```python
from build123d import *

# Parameters (mm, degrees)
F0_R     = 11
F1_DEPTH = 2.5
F2_SIZE  = 1.016
F3_R     = 8.25
F4_DEPTH = 0.5


with BuildPart() as f1:
    # F0 (on Top) → F1 (new body)
    with BuildSketch(Plane.XY):
        Circle(F0_R)
    extrude(amount=F1_DEPTH)

    # F2
    f2_edges = [f1.edges().sort_by_distance(p)[0] for p in [
        (-11, 0, 2.5),
    ]]
    chamfer(f2_edges, length=F2_SIZE)

    # F3 (on face) → F4 (cut)
    with BuildSketch(Plane(origin=(0, 0, 0), x_dir=(1, 0, 0), z_dir=(0, 0, -1))):
        Circle(F3_R)
    extrude(amount=-F4_DEPTH, mode=Mode.SUBTRACT)


solid = f1.part
```
Verification items for the finished model (mm, model axes). A direction names the side the tool comes from. Coordinates: 2 decimals unless noted, no trailing zeros. Loops run counter-clockwise (first coordinate to the right, second up) from the corner with the lowest first, then second, coordinate; pieces in that order, holes last. Notation, with made-up numbers: (81, -3) - (88, -3) arc R14 cw to (88, 6) - close; hole circle Ø4 at (33, 85.5). An arc over 180 degrees is marked (long way). Put each result on its own line as item: value.
Item 1: Section check C-C (z = 0.95). Enter the section's corners in (x, y).
Conclusion:
outline: circle Ø22 at (0, 0)
Item 2: Gauge pin test, flat ends, axial feed: pin 1 Ø1 at (x, z) = (4, 2) entering from +Y; pin 2 Ø1.5 at (x, z) = (-7.5, 1) entering from -Y; pin 3 Ø1.5 at (x, z) = (-8.5, 1.5) entering from +Y. Record the tip position at first contact, or that the pin passes through.
Conclusion:
pin 1: stops at y = 10.26
pin 2: stops at y = -8.69
pin 3: stops at y = 7.81
Item 3: Draft check along X on faces 3 (the face through (0, 0, 2.5)), 4 (the face through (0, 0, 0.5)), 5 (the face through (-2.38, -10.74, 0.73)). Enter one of: pulls with the +X half, pulls with the -X half, needs draft (parallel to the pull), parting line crosses it, or undercut.
Conclusion:
face 3: needs draft
face 4: undercut
face 5: parting line crosses it
Item 4: Section check A-A (y = 0). Enter the section's corners in (x, z), then the cut area to 3 significant figures.
Conclusion:
outline: (-11, 0) - (-8.25, 0) - (-8.25, 0.5) - (8.25, 0.5) - (8.25, 0) - (11, 0) - (11, 1.48) - (9.98, 2.5) - (-9.98, 2.5) - (-11, 1.48) - close
area: 45.7 mm2
Item 5: Set-up check for faces 1 (the face through (4, 7.4, 0)), 2 (the face through (7.62, 3.16, 0.25)): record each of +Z, -Z, +X, -X, +Y, -Y from which the full face is reachable in a straight line by a thin tool's end or side.
Conclusion:
face 1: -Z, +X, -X, +Y, -Y
face 2: -Z
Item 6: Scan lines: line 1 along Y through (x, z) = (0, 0.25); line 2 along Z through (x, y) = (7, 3); line 3 along X through (y, z) = (-0.25, 0.7). Record each from-to range of solid material in increasing order.
Conclusion:
line 1: y = -11 to -8.25, 8.25 to 11
line 2: z = 0.5 to 2.5
line 3: x = -11 to 11
Item 7: Section check D-D (z = 2.25). Enter the section's corners in (x, y).
Conclusion:
outline: circle Ø20.47 at (0, 0)
